```python
from build123d import *

# Parameters (mm, degrees)
F0_W     = 22.1742
F0_H     = 292.1
F1_DEPTH = 5.334
F2_W     = 5.334
F2_H     = 6.35
F3_DEPTH = 5.334
F5_DEPTH = 5.335
F6_W     = 5.08
F6_H     = 5.334
F7_DEPTH = 25.4
F8_W     = 22.1742
F8_H     = 2.54
F9_DEPTH = 25.4


with BuildPart() as f1:
    # F0 (on Front) → F1 (new body)
    with BuildSketch(Plane.XZ):
        with Locations((-23.465344, 68.295897)):
            Rectangle(F0_W, F0_H)
    extrude(amount=F1_DEPTH)

    # F2 (on face) → F3 (join)
    with BuildSketch(Plane.YZ.offset(-12.378244)):
        with Locations((-2.667, 165.704897)):
            Rectangle(F2_W, F2_H)
        with Locations((-2.667, 68.295897)):
            Rectangle(F2_W, F2_H)
        with Locations((-2.667, -29.113103)):
            Rectangle(F2_W, F2_H)
    extrude(amount=F3_DEPTH)

    # F4 (on face) → F5 (cut, through all)
    with BuildSketch(Plane.XZ.offset(5.334)):
        Polygon((-26.043444, -71.404103), (-26.043444, -77.754103), (-22.741444, -77.754103), (-22.741444, -71.404103), (-21.598444, -71.404103), (-21.598444, -69.118103), (-22.741444, -69.118103), (-22.741444, -65.054103), (-26.043444, -65.054103), (-26.043444, -69.118103), (-27.186444, -69.118103), (-27.186444, -71.404103), align=None)
        Polygon((-26.043444, 214.345897), (-26.043444, 207.995897), (-27.186444, 207.995897), (-27.186444, 205.709897), (-26.043444, 205.709897), (-26.043444, 201.645897), (-22.741444, 201.645897), (-22.741444, 205.709897), (-21.598444, 205.709897), (-21.598444, 207.995897), (-22.741444, 207.995897), (-22.741444, 214.345897), align=None)
    extrude(amount=-F5_DEPTH, mode=Mode.SUBTRACT)

    # F6 (on face) → F7 (cut)
    with BuildSketch(Plane.XZ.offset(5.334)):
        with Locations((-14.918244, 159.862897)):
            Rectangle(F6_W, F6_H)
        with Locations((-14.918244, 62.453897)):
            Rectangle(F6_W, F6_H)
        with Locations((-14.918244, -34.955103)):
            Rectangle(F6_W, F6_H)
    extrude(amount=-F7_DEPTH, mode=Mode.SUBTRACT)

    # F8 (on face) → F9 (cut)
    with BuildSketch(Plane.XZ.offset(5.334)):
        with Locations((-23.465344, 213.075897)):
            Rectangle(F8_W, F8_H)
        with Locations((-23.465344, -76.484103)):
            Rectangle(F8_W, F8_H)
    extrude(amount=-F9_DEPTH, mode=Mode.SUBTRACT)


solid = f1.part
```
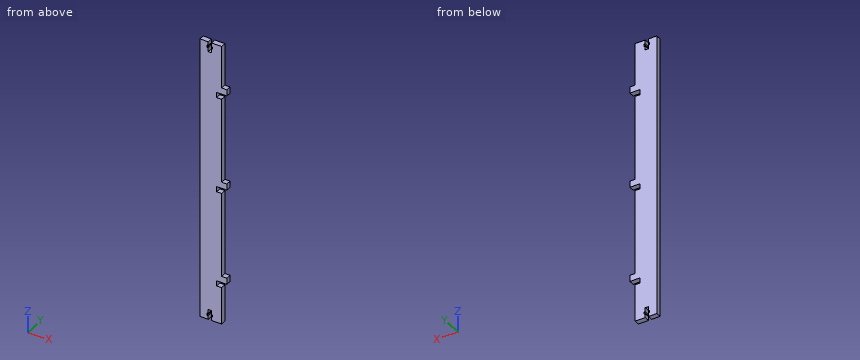
Can you work these out from the model? Positions are in its coordinate system, mm. Coordinates: 2 decimals unless noted, no trailing zeros. Order: outer loops, then holes, each group sorted by start corner. A loop starts at its lowest first (then second) coordinate and runs counter-clockwise, first axis right, second up. Notation, with made-up numbers: (32.5, 65.5) - (46.5, 65.5) arc R22 cw to (46.5, 88.5) - close; hole circle Ø6 at (85, -21). An arc over 180 degrees is marked (long way). Answer in a Markdown table with one row per item.
1. If I drill on line 1 along Z through (x, y) = (-14, -3.45); line 2 along Z through (x, y) = (-11.75, -3.6); line 3 along X through (y, z) = (-0.9, 26), over which ranges is the centre line in solid material (lowest first)?
Reply:
| item | result |
|---|---|
| line 1 | z = -75.21 to -37.62, -32.29 to 59.79, 65.12 to 157.2, 162.53 to 211.81 |
| line 2 | z = -32.29 to -25.94, 65.12 to 71.47, 162.53 to 168.88 |
| line 3 | x = -34.55 to -12.38 |
2. For pin 1 (2.5 mm diameter, centred on x = -10, y = -2, fed in from -Z); pin 2 (1.1 mm diameter, centred on y = -1.5, z = -70, fed in from +X); pin 3 (2.5 mm diameter, centred on y = -2.5, z = -35, fed in from +X), each with a flat end and sliding along its axis, tell me the tip position at first contact or that it passes through.
Reply:
| item | result |
|---|---|
| pin 1 | stops at z = -32.29 |
| pin 2 | stops at x = -12.38 |
| pin 3 | stops at x = -17.46 |
3. Suppose I cut it at A-A (z = 12.5). Please give me the cut outline in (x, y), and give its area (3 significant figures).
Reply:
| item | result |
|---|---|
| outline | (-34.55, -5.33) - (-12.38, -5.33) - (-12.38, 0) - (-34.55, 0) - close |
| area | 118 mm^2 |
